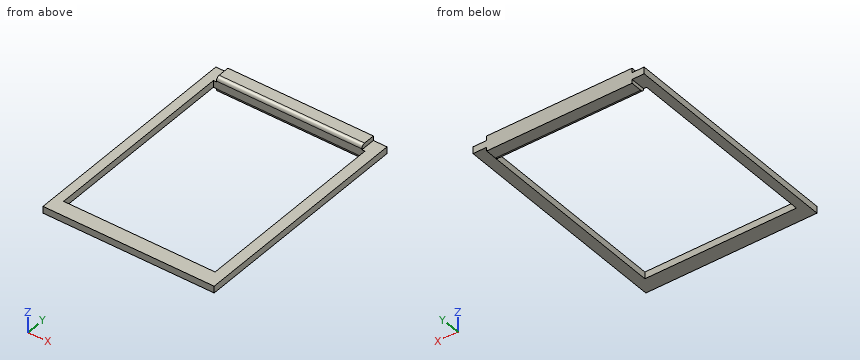
from build123d import *

# Parameters (mm, degrees)
SKETCH2_W                = 56.5
SKETCH2_H                = 75
SKETCH2_W_2              = 50
SKETCH2_H_2              = 65
BOSS_EXTRUDE1_DEPTH      = 2.25
SKETCH3_W                = 48
SKETCH3_H                = 5
BOSS_EXTRUDE2_DEPTH      = 1.5
SKETCH3_4_W              = 48
SKETCH3_4_H              = 5
BOSS_EXTRUDE3_DEPTH      = 1.5
BOSS_EXTRUDE3_DEPTH_BACK = 3.5
FILLET3_R                = 1.2


with BuildPart() as part:
    # Sketch2 → Boss-Extrude1 (new body)
    with BuildSketch(Plane.XY):
        with Locations((28.25, 37.5)):
            Rectangle(SKETCH2_W, SKETCH2_H)
        with Locations((28, 37.5)):
            Rectangle(SKETCH2_W_2, SKETCH2_H_2, mode=Mode.SUBTRACT)
    extrude(amount=BOSS_EXTRUDE1_DEPTH)

    # Sketch3 → Boss-Extrude2 (add)
    with BuildSketch(Plane.XY.offset(2.25)):
        with Locations((28, 72.5)):
            Rectangle(SKETCH3_W, SKETCH3_H)
    extrude(amount=BOSS_EXTRUDE2_DEPTH)

    # Sketch3_4 → Boss-Extrude3 (add, two sides)
    with BuildSketch(Plane.XY.offset(2.25)) as boss_extrude3_sk:
        with Locations((28, 72.5)):
            Rectangle(SKETCH3_4_W, SKETCH3_4_H)
    extrude(amount=BOSS_EXTRUDE3_DEPTH)
    extrude(boss_extrude3_sk.sketch, amount=-BOSS_EXTRUDE3_DEPTH_BACK)

    # Fillet3
    fillet3_edges = [part.edges().sort_by_distance(p)[0] for p in [
        (28, 70, 3.75),
        (28, 70, -1.25),
    ]]
    fillet(fillet3_edges, radius=FILLET3_R)


solid = part.part
Here's how the part is built. I have some questions about the finished solid (model axes, mm). Coordinates: 2 decimals unless noted, no trailing zeros. Write each loop counter-clockwise with the first axis right and the second up, starting at its lowest first coordinate (ties: lowest second). Pieces come first, ordered by that corner, then holes.
1) If we section it at C-C (z = 1.05): List the corners of the cut face in (x, y) for me.
Filled in:
outline: (0, 0) - (56.5, 0) - (56.5, 75) - (0, 75) - close; hole (3, 5) - (53, 5) - (53, 70) - (3, 70) - close
2) If I drill on line 1 (Y direction, x = 33, z = 0.25); line 2 (X direction, y = 45.5, z = 1.85); line 3 (Y direction, x = 40, z = -0.1), over which ranges is the centre line in solid material (lowest first)?
Filled in:
line 1: y = 0 to 5, 70 to 75
line 2: x = 0 to 3, 53 to 56.5
line 3: y = 70 to 75
3) If we section it at A-A (y = 37): List the corners of the cut face in (x, z) for me.
Filled in:
outline: (0, 0) - (3, 0) - (3, 2.25) - (0, 2.25) - close; (53, 0) - (56.5, 0) - (56.5, 2.25) - (53, 2.25) - close
4) I'm going to push flat-ended pins straight in: pin 1 (1.2 mm diameter, centred on y = 73, z = 3, fed in from +X); pin 2 (12 mm diameter, centred on x = 48.5, y = 21.5, fed in from +Z). Where does each tip first touch, or does it pass through?
Filled in:
pin 1: stops at x = 52
pin 2: stops at z = 2.25
5) If we section it at B-B (x = 37): List the corners of the cut face in (y, z) for me.
Filled in:
outline: (0, 0) - (5, 0) - (5, 2.25) - (0, 2.25) - close; (70, -0.05) arc R1.2 ccw to (71.2, -1.25) - (75, -1.25) - (75, 3.75) - (71.2, 3.75) arc R1.2 ccw to (70, 2.55) - close
